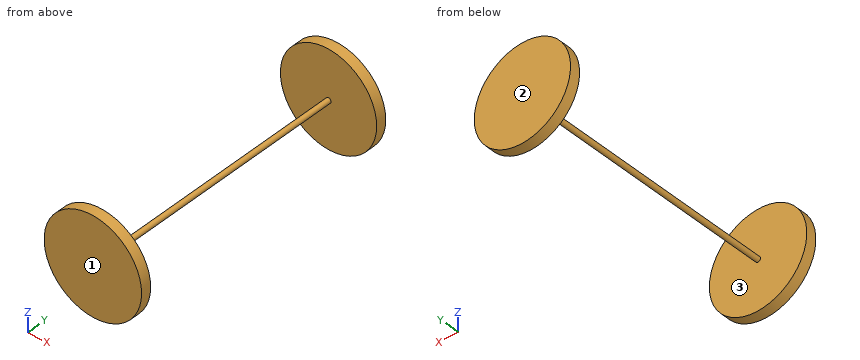
```python
from build123d import *

# Parameters (mm, degrees)
F0_R     = 0.5
F1_DEPTH = 50
F3_R     = 9.458043
F4_DEPTH = 2
F6_R     = 9.572507
F7_DEPTH = 2


with BuildPart() as f1:
    # F0 (on Front) → F1 (new body)
    with BuildSketch(Plane.XZ):
        with Locations((0, 8.707933)):
            Circle(F0_R)
    extrude(amount=F1_DEPTH)

    # F3 (on Front) → F4 (join)
    with BuildSketch(Plane.XZ):
        with Locations((0, 8.897236)):
            Circle(F3_R)
    extrude(amount=-F4_DEPTH)

    # F6 (on offset) → F7 (join)
    with BuildSketch(Plane.XZ.offset(50)):
        with Locations((0, 8.626235)):
            Circle(F6_R)
    extrude(amount=F7_DEPTH)


solid = f1.part
```
Part model, mm, in its own coordinate system. Face numbers are marked on the shaded views. Give positions to 0.01 mm unless a question says otherwise; leave off trailing zeros. Loops run counter-clockwise (first coordinate to the right, second up) from the corner with the lowest first, then second, coordinate; pieces in that order, holes last. Notation, with made-up numbers: M 63,44.25 L 101,44.25 A14 cw 101,59.25 Z; hole C 74,-28.75 d2. An arc over 180 degrees is marked long. Return JSON: item names as keys, results as strings.
1) Pull direction Y, two halves, no side cores. Call the marked faces 1, 2 and 3: released by +Y, released by -Y, zero draft, split by the parting line, or undercut.
Calculated:
{"face 1": "released by -Y", "face 2": "released by +Y", "face 3": "undercut"}
2) Saw through at C-C, the plane x = 0. List the corners of the cut face in (y, z).
Calculated:
{"outline": "M -52,-0.95 L -50,-0.95 L -50,8.21 L 0,8.21 L 0,-0.56 L 2,-0.56 L 2,18.36 L 0,18.36 L 0,9.21 L -50,9.21 L -50,18.2 L -52,18.2 Z"}
3) Saw through at B-B, the plane z = 15.25. List the corners of the cut face in (x, y).
Calculated:
{"outline": "M -7.01,0 L 7.01,0 L 7.01,2 L -7.01,2 Z; M -6.91,-52 L 6.91,-52 L 6.91,-50 L -6.91,-50 Z"}
4) Saw through at A-A, the plane x = 4.5. List the corners of the cut face in (y, z).
Calculated:
{"outline": "M -52,0.18 L -50,0.18 L -50,17.08 L -52,17.08 Z; M 0,0.58 L 2,0.58 L 2,17.22 L 0,17.22 Z"}
5) Drill centre lines: line 1 (Y direction, x = 5.5, z = 11.5); line 2 (X direction, y = -11, z = 8.5). Where is each one in solid material? Low to high.
Calculated:
{"line 1": "y = -52 to -50, 0 to 2", "line 2": "x = -0.45 to 0.45"}
6) Flat gauge pins, fed straight in: pin 1 Ø2 at (y, z) = (-30.5, 10) entering from +X; pin 2 Ø5 at (x, y) = (1, -33.5) entering from -Z. Where does each tip first touch, or does it go through?
Calculated:
{"pin 1": "stops at x = 0.41", "pin 2": "stops at z = 8.21"}
7) Saw through at D-D, the plane y = -21. List the corners of the cut face in (x, z).
Calculated:
{"outline": "C 0,8.71 d1"}
